from build123d import *

# Parameters (mm, degrees)
SKETCH1_R           = 3.65
SKETCH1_R_2         = 2.4
BOSS_EXTRUDE1_DEPTH = 7.7
SKETCH2_R           = 3.15
SKETCH2_R_2         = 2.4
CUT_EXTRUDE1_DEPTH  = 0.5
SKETCH4_R           = 2.9
BOSS_EXTRUDE2_DEPTH = 5.7
SKETCH5_R           = 2.25
BOSS_EXTRUDE3_DEPTH = 10.2
SKETCH8_R           = 2.4
CUT_EXTRUDE5_DEPTH  = 8.2000001
SKETCH14_R          = 2.45
SKETCH14_R_2        = 2.25
BOSS_EXTRUDE5_DEPTH = 0.2
SKETCH10_R          = 1.5
CUT_EXTRUDE6_DEPTH  = 8.35
SKETCH7_W           = 1
SKETCH7_H           = 5.978668982
CUT_EXTRUDE7_DEPTH  = 1.7


with BuildPart() as part:
    # Sketch1 → Boss-Extrude1 (new body)
    with BuildSketch(Plane(origin=(0, 0, 0), x_dir=(1, 0, 0), z_dir=(0, 1, 0))):
        Circle(SKETCH1_R)
        Circle(SKETCH1_R_2, mode=Mode.SUBTRACT)
    extrude(amount=BOSS_EXTRUDE1_DEPTH)

    # Sketch2 → Cut-Extrude1 (cut)
    with BuildSketch(Plane(origin=(0, 7.7, 0), x_dir=(1, 0, 0), z_dir=(0, 1, 0))):
        Circle(SKETCH2_R)
        Circle(SKETCH2_R_2, mode=Mode.SUBTRACT)
    extrude(amount=-CUT_EXTRUDE1_DEPTH, mode=Mode.SUBTRACT)

    # Sketch4 → Boss-Extrude2 (add)
    with BuildSketch(Plane.XY):
        with Locations((0, 3.85)):
            Circle(SKETCH4_R)
    extrude(amount=BOSS_EXTRUDE2_DEPTH)

    # Sketch5 → Boss-Extrude3 (add)
    with BuildSketch(Plane.XY):
        with Locations((0, 3.85)):
            Circle(SKETCH5_R)
    extrude(amount=BOSS_EXTRUDE3_DEPTH)

    # Sketch8 → Cut-Extrude5 (cut, through all)
    with BuildSketch(Plane(origin=(0, 7.2, 0), x_dir=(1, 0, 0), z_dir=(0, 1, 0))):
        Circle(SKETCH8_R)
    extrude(amount=-CUT_EXTRUDE5_DEPTH, mode=Mode.SUBTRACT)

    # Sketch14 → Boss-Extrude5 (add)
    with BuildSketch(Plane.XY.offset(10)):
        with Locations((0, 3.85)):
            Circle(SKETCH14_R)
        with Locations((0, 3.85)):
            Circle(SKETCH14_R_2, mode=Mode.SUBTRACT)
    extrude(amount=BOSS_EXTRUDE5_DEPTH)

    # Sketch10 → Cut-Extrude6 (cut, through all)
    with BuildSketch(Plane.XY.offset(2.85)):
        with Locations((0, 3.85)):
            Circle(SKETCH10_R)
    extrude(amount=CUT_EXTRUDE6_DEPTH, mode=Mode.SUBTRACT)

    # Sketch7 → Cut-Extrude7 (cut)
    with BuildSketch(Plane.XY.offset(10.2)):
        with Locations((0, 3.85)):
            Rectangle(SKETCH7_W, SKETCH7_H)
    extrude(amount=-CUT_EXTRUDE7_DEPTH, mode=Mode.SUBTRACT)


solid = part.part
The model under review builds one solid part; all positions refer to its coordinate system, in mm. A direction names the side the tool comes from. Give positions to 0.01 mm unless a question says otherwise; leave off trailing zeros. Loops run counter-clockwise (first coordinate to the right, second up) from the corner with the lowest first, then second, coordinate; pieces in that order, holes last. Notation, with made-up numbers: (-27.5, -1.5) -> (-5.5, -1.5) arc R6 cw to (-5.5, 3.5) -> close; hole circle Ø6 at (53.5, 10.25). An arc over 180 degrees is marked (long way). Answer as a JSON object with one key per item and string values. Group by question number.
Q1. Insertion check: pin 1 (0.5 mm diameter, centred on y = 2, z = 9, fed in from +X); pin 2 (0.9 mm diameter, centred on x = 0, y = 2, fed in from +Z); pin 3 (2 mm diameter, centred on y = 2, z = 4.5, fed in from -X). Each pin has a flat end and moves straight along its axis. Give the tip position at first contact, or say it passes through.
Q2. Wall thickness on line 1 along X through (y, z) = (5.5, 0); line 2 along X through (y, z) = (3.75, 7.5); line 3 along Y through (x, z) = (0, 6): over which ranges is each line inside the solid? List them lowest first.
Q3. Take a section at D-D (z = 8). Write out the cut boundary in (x, y), plus the area to 3 significant figures.
Q4. Draft analysis for pull direction Z (two halves, no side actions). For faces 6 (the flat face through (0.5, 2, 9)), 7 (the cylindrical face through (2.146, 4.526, 7.82)), 8 (the flat face through (2, 4, 10.2)), state which applies: pulls with the +Z half, pulls with the -Z half, needs draft (parallel to the pull), parting line crosses it, or undercut.
Q5. Tool access review of faces 1 (the flat face through (-2, 4, 10.2)), 2 (the cylindrical face through (1.29, 3.55, -2.024)), 3 (the flat face through (0.5, 5.6, 9.4)), 4 (the cylindrical face through (-2.5, 7.454, 1.917)), 5 (the cylindrical face through (1.386, 3.275, 6.474)): name each direction out of +Z, -Z, +X, -X, +Y, -Y from which nothing blocks a thin tool from reaching the whole face with its end or side.
Q6. Take a section at C-C (z = 0). Write out the cut boundary in (x, y), plus the area to 3 significant figures.
Q7. Take a section at A-A (x = 0). Write out the cut boundary in (y, z), plus the area to 3 significant figures.
Q8. Take a section at B-B (y = 3.85). Write out the cut boundary in (x, z), plus the area to 3 significant figures.
Answer below:
{
 "1": {"pin 1": "stops at x = 1.58", "pin 2": "stops at z = 8.5", "pin 3": "stops at x = -2.77"},
 "2": {"line 1": "x = -3.65 to -2.4, 2.4 to 3.65", "line 2": "x = -2.25 to -1.5, 1.5 to 2.25", "line 3": "y = 1.6 to 2.35, 5.35 to 6.1"},
 "3": {"outline": "circle Ø4.5 at (0, 3.85); hole circle Ø3 at (0, 3.85)", "area": "8.84 mm2"},
 "4": {"face 6": "needs draft", "face 7": "undercut", "face 8": "pulls with the +Z half"},
 "5": {"face 1": "+Z, +X, -X, +Y, -Y", "face 2": "+Y, -Y", "face 3": "+Z, +Y, -Y", "face 4": "+Y", "face 5": "+Z"},
 "6": {"outline": "(-3.65, 0) -> (-2.4, 0) -> (-2.4, 7.2) -> (-3.15, 7.2) -> (-3.15, 7.7) -> (-3.65, 7.7) -> close; (2.4, 0) -> (3.65, 0) -> (3.65, 7.7) -> (3.15, 7.7) -> (3.15, 7.2) -> (2.4, 7.2) -> close", "area": "18.5 mm2"},
 "7": {"outline": "(0, -3.65) -> (7.7, -3.65) -> (7.7, -3.15) -> (7.2, -3.15) -> (7.2, -2.4) -> (0, -2.4) -> close; (0, 2.4) -> (7.2, 2.4) -> (7.2, 3.15) -> (7.7, 3.15) -> (7.7, 3.65) -> (6.75, 3.65) -> (6.75, 5.7) -> (6.1, 5.7) -> (6.1, 8.5) -> (5.35, 8.5) -> (5.35, 2.85) -> (2.35, 2.85) -> (2.35, 8.5) -> (1.6, 8.5) -> (1.6, 5.7) -> (0.95, 5.7) -> (0.95, 3.65) -> (0, 3.65) -> close", "area": "26.0 mm2"},
 "8": {"outline": "(-2.9, 2.22) arc R3.65 ccw (long way) to (2.9, 2.22) -> (2.9, 5.7) -> (2.25, 5.7) -> (2.25, 10) -> (2.45, 10) -> (2.45, 10.2) -> (1.5, 10.2) -> (1.5, 2.85) -> (-1.5, 2.85) -> (-1.5, 10.2) -> (-2.45, 10.2) -> (-2.45, 10) -> (-2.25, 10) -> (-2.25, 5.7) -> (-2.9, 5.7) -> close; hole circle Ø4.8 at (0, 0)", "area": "36.4 mm2"}
}
